The model under review builds one solid part; all positions refer to its coordinate system, in mm. Face numbers are marked on the shaded views. A direction names the side the tool comes from. Round coordinates to 2 decimals unless told otherwise and drop trailing zeros. Loops run counter-clockwise (first coordinate to the right, second up) from the corner with the lowest first, then second, coordinate; pieces in that order, holes last. Notation, with made-up numbers: M 54.5,-4.5 L 74.5,-4.5 A8 ccw 74.5,7.5 Z; hole C -38.75,-19 d6. An arc over 180 degrees is marked long. Answer in a Markdown table with one row per item. Add a question column.
from build123d import *

# Parameters (mm, degrees)
SKETCH_1_R               = 14
EXTRUDE_1_DEPTH          = 4
CUT_EXTRUDE_1_DEPTH      = 4
PATTERN_CIRCULAR_1_COUNT = 26
CUT_EXTRUDE_2_REACH      = 6
SKETCH_3_R               = 3
SKETCH_3_R_2             = 1.6


with BuildPart() as part:
    # 草圖1 → 填料-伸長1 (new body)
    with BuildSketch(Plane.XY):
        Circle(SKETCH_1_R)
    extrude(amount=EXTRUDE_1_DEPTH)

    # 草圖2 → 除料-伸長1 (cut)
    with BuildSketch(Plane.XY.offset(4)):
        with BuildLine():
            ThreePointArc((-1.421594657, 13.927636865), (0, 14), (1.421594657, 13.927636865))
            ThreePointArc((1.421594657, 13.927636865), (0.822322703, 12.888806427), (0.476978653, 11.74031479))
            ThreePointArc((0.476978653, 11.74031479), (0, 11.75), (-0.476978653, 11.74031479))
            ThreePointArc((-0.476978653, 11.74031479), (-0.822322703, 12.888806427), (-1.421594657, 13.927636865))
        make_face()
    cut_extrude_1 = extrude(amount=-CUT_EXTRUDE_1_DEPTH, mode=Mode.SUBTRACT)

    # 環狀複製排列1: 除料-伸長1 ×26 about axis
    pattern_circular_1_axis = Axis((0, 0, 0), (0, 0, 1))
    for i in range(1, PATTERN_CIRCULAR_1_COUNT):
        add(cut_extrude_1.rotate(pattern_circular_1_axis, i * 360 / PATTERN_CIRCULAR_1_COUNT), mode=Mode.SUBTRACT)

    # 草圖3 → 除料-伸長2 (cut, up to next)
    with BuildSketch(Plane.XY.offset(4), mode=Mode.PRIVATE) as cut_extrude_2_sk1:
        Circle(SKETCH_3_R)
    cut_extrude_2_tool1 = extrude(cut_extrude_2_sk1.sketch, amount=-CUT_EXTRUDE_2_REACH, mode=Mode.PRIVATE) & part.part
    add(cut_extrude_2_tool1.solids().sort_by_distance((0, 0, 4))[0], mode=Mode.SUBTRACT)
    # 草圖3 → 除料-伸長2 (cut, up to next)
    with BuildSketch(Plane.XY.offset(4), mode=Mode.PRIVATE) as cut_extrude_2_sk2:
        with Locations((0, 7)):
            Circle(SKETCH_3_R_2)
    cut_extrude_2_tool2 = extrude(cut_extrude_2_sk2.sketch, amount=-CUT_EXTRUDE_2_REACH, mode=Mode.PRIVATE) & part.part
    add(cut_extrude_2_tool2.solids().sort_by_distance((0, 7, 4))[0], mode=Mode.SUBTRACT)
    # 草圖3 → 除料-伸長2 (cut, up to next)
    with BuildSketch(Plane.XY.offset(4), mode=Mode.PRIVATE) as cut_extrude_2_sk3:
        with Locations((7, 0)):
            Circle(SKETCH_3_R_2)
    cut_extrude_2_tool3 = extrude(cut_extrude_2_sk3.sketch, amount=-CUT_EXTRUDE_2_REACH, mode=Mode.PRIVATE) & part.part
    add(cut_extrude_2_tool3.solids().sort_by_distance((7, 0, 4))[0], mode=Mode.SUBTRACT)
    # 草圖3 → 除料-伸長2 (cut, up to next)
    with BuildSketch(Plane.XY.offset(4), mode=Mode.PRIVATE) as cut_extrude_2_sk4:
        with Locations((0, -7)):
            Circle(SKETCH_3_R_2)
    cut_extrude_2_tool4 = extrude(cut_extrude_2_sk4.sketch, amount=-CUT_EXTRUDE_2_REACH, mode=Mode.PRIVATE) & part.part
    add(cut_extrude_2_tool4.solids().sort_by_distance((0, -7, 4))[0], mode=Mode.SUBTRACT)
    # 草圖3 → 除料-伸長2 (cut, up to next)
    with BuildSketch(Plane.XY.offset(4), mode=Mode.PRIVATE) as cut_extrude_2_sk5:
        with Locations((-7, 0)):
            Circle(SKETCH_3_R_2)
    cut_extrude_2_tool5 = extrude(cut_extrude_2_sk5.sketch, amount=-CUT_EXTRUDE_2_REACH, mode=Mode.PRIVATE) & part.part
    add(cut_extrude_2_tool5.solids().sort_by_distance((-7, 0, 4))[0], mode=Mode.SUBTRACT)


solid = part.part
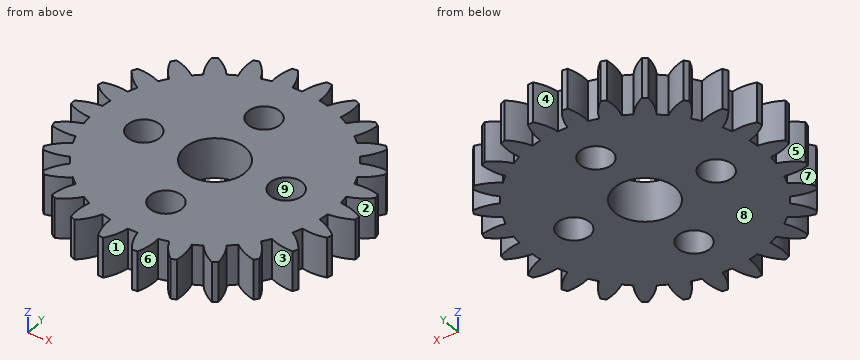
1. To check wall thickness, follow probe 1 along Y at (x, z) = (0, 2.35); probe 2 along X at (y, z) = (10.75, 3); probe 3 along Y at (x, z) = (1, 0.4). State the ranges of each line that lie inside material, in increasing order.
2. Machinability: for the marked faces 1, 2, 3, 4 and 5, which of the approach directions +Z, -Z, +X, -X, +Y, -Y give a long, thin tool a straight path to every point of the face, cutting with its end or side? Answer none if there is none.
3. Take a section at B-B, the plane x = 7. State the section outline as (y, z) points, and give its area (3 significant figures).
4. Mouldability with a two-part tool opening along X and no side actions: class the marked faces 6, 7, 8 and 9 as released by +X, released by -X, zero draft, split by the parting line, or undercut.
5. For pin 1 Ø1.9 at (x, y) = (0, 7) entering from +Z; pin 2 Ø1 at (y, z) = (1, 3) entering from +X, all flat-tipped, find the tip position at first contact; note any pin that passes through.
6. Take a section at A-A, the plane x = 0. State the section outline as (y, z) points, and give its area (3 significant figures).
7. Take a section at C-C, the plane z = 0.6. State how many separate pieces and enclosed holes the cut face has, and give its area (3 significant figures).
Check sheet entries:
| question | item | result |
|---|---|---|
| 1 | probe 1 | y = -11.75 to -8.6, -5.4 to -3, 3 to 5.4, 8.6 to 11.75 |
| 1 | probe 2 | x = -8.08 to -6.4, -5.07 to 5.07, 6.4 to 8.08 |
| 1 | probe 3 | y = -13.26 to -8.25, -5.75 to -2.83, 2.83 to 5.75, 8.25 to 13.26 |
| 2 | face 1 | +Z, -Z, -Y |
| 2 | face 2 | +Z, -Z, +X |
| 2 | face 3 | +Z, -Z |
| 2 | face 4 | +Z, -Z, +Y |
| 2 | face 5 | +Z, -Z, -X |
| 3 | outline | M -11.24,0 L -1.6,0 L -1.6,4 L -11.24,4 Z; M 1.6,0 L 11.24,0 L 11.24,4 L 1.6,4 Z |
| 3 | area | 77.1 mm^2 |
| 4 | face 6 | undercut |
| 4 | face 7 | released by -X |
| 4 | face 8 | zero draft |
| 4 | face 9 | undercut |
| 5 | pin 1 | passes through |
| 5 | pin 2 | stops at x = 13.54 |
| 6 | outline | M -11.75,0 L -8.6,0 L -8.6,4 L -11.75,4 Z; M -5.4,0 L -3,0 L -3,4 L -5.4,4 Z; M 3,0 L 5.4,0 L 5.4,4 L 3,4 Z; M 8.6,0 L 11.75,0 L 11.75,4 L 8.6,4 Z |
| 6 | area | 44.4 mm^2 |
| 7 | separate pieces | 1 |
| 7 | enclosed holes | 5 |
| 7 | area | 455 mm^2 |
